Autodesk Inventor part; units mm, degrees
ref_plane "YZ Plane" through (0, 0, 0) normal (1, 0, 0) x (0, 1, 0)
ref_plane "XZ Plane" through (0, 0, 0) normal (0, 1, 0) x (-1, 0, 0)
ref_plane "XY Plane" through (0, 0, 0) normal (0, 0, 1) x (1, 0, 0)
sketch "Sketch1" plane through (0, 0, 0) normal (0, 0, 1) x (1, 0, 0)
  line L0 (0, 0) -> (21, 0)
  line L1 (21, 0) -> (21, 39)
  line L2 (21, 39) -> (0, 39)
  line L3 (0, 39) -> (0, 0)
  dimension "d0" = 21
  dimension "d1" = 39
extrude "Extrusion1" add sketch "Sketch1" along normal blind 9
sketch "Sketch2" plane through (21, 39, 0) normal (0, 1, 0) x (0, 0, -1)
  line L0 (0, 0) -> (-9, 0)
  circle A0 centre (-4.5, 3) radius 0.75
  circle A1 centre (-4.5, 4.5) radius 0.75
  circle A2 centre (-4.5, 16.5) radius 0.75
  circle A3 centre (-4.5, 18) radius 0.75
  line L1 (0, 21) -> (-9, 21)
  point P0 (-4.5, 0)
  point P1 (-4.5, 0)
  point P2 (-4.5, 0)
  point P3 (-4.5, 17.25)
  point P4 (-4.5, 3.75)
  dimension "d14" = 1.5
  dimension "d15" = 1.5
  dimension "d16" = 1.5
  dimension "d17" = 3
  dimension "d18" = 3
extrude "Extrusion2" add sketch "Sketch2" along normal blind 12
sketch "Sketch3" plane through (0, 0, 0) normal (0, -1, 0) x (0, 0, 1)
  circle A0 centre (4.5, -18) radius 0.75
  circle A1 centre (4.5, -16.5) radius 0.75
  circle A2 centre (4.5, -15) radius 0.75
  line L0 (0, -21) -> (9, -21)
  point P0 (4.5, -21)
  point P1 (4.5, -15.75)
  point P2 (4.5, -17.25)
  dimension "d19" = 1.5
  dimension "d20" = 1.5
  dimension "d21" = 1.5
  dimension "d22" = 3
extrude "Extrusion3" add sketch "Sketch3" along normal blind 12
equation "\"d21\" = d20"
properties part number "Brushed ESC"
The model under review builds one solid part; all positions refer to its coordinate system, in mm. Round coordinates to 2 decimals unless told otherwise and drop trailing zeros. Order: outer loops, then holes, each group sorted by start corner. A loop starts at its lowest first (then second) coordinate and runs counter-clockwise, first axis right, second up. Notation, with made-up numbers: M 37,3.5 L 47,3.5 A22 cw 47,19.5 Z; hole C 23.5,0 d5. An arc over 180 degrees is marked long. Use a Markdown table: item, result.
1) Wall thickness on line 1 along Y through (x, z) = (3.5, 1.5): over which ranges is the line inside the solid? List them lowest first. Write a range as [from, to].
Report:
| item | result |
|---|---|
| line 1 | [0, 39] |
2) Insertion check: pin 1 (5 mm diameter, centred on x = 10, y = -4, fed in from +Z); pin 2 (4.5 mm diameter, centred on x = 6.5, z = 4.5, fed in from -Y); pin 3 (3 mm diameter, centred on y = 43, z = 3.5, fed in from -X); pin 4 (4.5 mm diameter, centred on x = 11.5, z = 6.5, fed in from +Y). Each pin has a flat end and moves straight along its axis. Give the tip position at first contact, or say it passes through.
Report:
| item | result |
|---|---|
| pin 1 | through |
| pin 2 | y = 0 |
| pin 3 | x = 2.25 |
| pin 4 | y = 39 |
3) Consider section B-B (x = 12.5). Write out the cut boundary in (y, z).
Report:
| item | result |
|---|---|
| outline | M 0,0 L 39,0 L 39,9 L 0,9 Z |
4) Consider section C-C (z = 8.25). Write out the cut boundary in (x, y).
Report:
| item | result |
|---|---|
| outline | M 0,0 L 21,0 L 21,39 L 0,39 Z |
